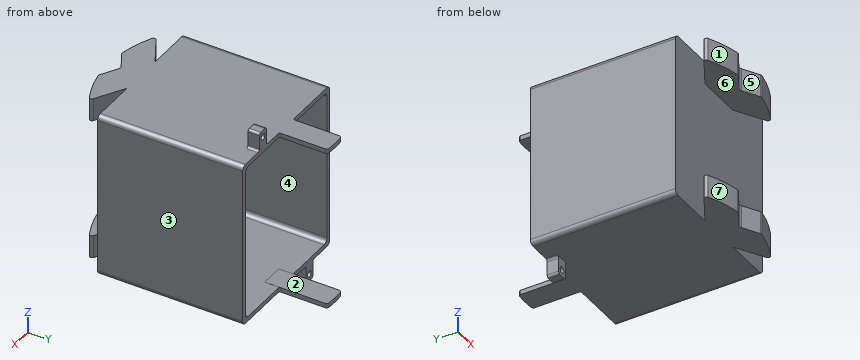
from build123d import *

# Parameters (mm, degrees)
BOSS_EXTRUDE1_DEPTH = 70
CUT_EXTRUDE1_DEPTH  = 79.756
BOSS_EXTRUDE3_DEPTH = 2.54
BOSS_EXTRUDE4_DEPTH = 2.54
BOSS_EXTRUDE5_DEPTH = 12.7
BOSS_EXTRUDE6_START = -2.54
BOSS_EXTRUDE6_DEPTH = 2.54
BOSS_EXTRUDE7_START = -12.7
BOSS_EXTRUDE7_DEPTH = 12.7
BOSS_EXTRUDE8_DEPTH = 8
SKETCH9_R           = 1.685173155
BOSS_EXTRUDE9_DEPTH = 6.35
FILLET1_R           = 1.27
FILLET3_R           = 1


# Read off the part's stored shape, not the designer's step: Boss-Extrude8
with BuildPart() as part:
    # Sketch1 → Boss-Extrude1 (new body)
    with BuildSketch(Plane(origin=(0, 0, 0), x_dir=(1, 0, 0), z_dir=(0, 1, 0))):
        with BuildLine():
            Line((-36.96, -46), (36.96, -46))
            ThreePointArc((36.96, -46), (38.756051224, -45.256051224), (39.5, -43.46))
            Line((39.5, -43.46), (39.5, 43.46))
            ThreePointArc((39.5, 43.46), (38.756051224, 45.256051224), (36.96, 46))
            Line((36.96, 46), (-36.96, 46))
            ThreePointArc((-36.96, 46), (-38.756051224, 45.256051224), (-39.5, 43.46))
            Line((-39.5, 43.46), (-39.5, -43.46))
            ThreePointArc((-39.5, -43.46), (-38.756051224, -45.256051224), (-36.96, -46))
        make_face()
    extrude(amount=-BOSS_EXTRUDE1_DEPTH)

    # Sketch2 → Cut-Extrude1 (cut)
    with BuildSketch(Plane(origin=(0, 0, 0), x_dir=(1, 0, 0), z_dir=(0, 1, 0))):
        with BuildLine():
            Line((-34.46, -43.5), (34.46, -43.5))
            ThreePointArc((34.46, -43.5), (36.256051224, -42.756051224), (37, -40.96))
            Line((37, -40.96), (37, 40.96))
            ThreePointArc((37, 40.96), (36.256051224, 42.756051224), (34.46, 43.5))
            Line((34.46, 43.5), (-34.46, 43.5))
            ThreePointArc((-34.46, 43.5), (-36.256051224, 42.756051224), (-37, 40.96))
            Line((-37, 40.96), (-37, -40.96))
            ThreePointArc((-37, -40.96), (-36.256051224, -42.756051224), (-34.46, -43.5))
        make_face()
    extrude(amount=-CUT_EXTRUDE1_DEPTH, mode=Mode.SUBTRACT)

    # Sketch4 → Boss-Extrude3 (add)
    with BuildSketch(Plane.XZ.offset(70)):
        with BuildLine():
            Line((36.96, 46), (-36.96, 46))
            ThreePointArc((-36.96, 46), (-38.756051224, 45.256051224), (-39.5, 43.46))
            Line((-39.5, 43.46), (-39.5, -43.46))
            ThreePointArc((-39.5, -43.46), (-38.756051224, -45.256051224), (-36.96, -46))
            Line((-36.96, -46), (36.96, -46))
            ThreePointArc((36.96, -46), (38.756051224, -45.256051224), (39.5, -43.46))
            Line((39.5, -43.46), (39.5, 43.46))
            ThreePointArc((39.5, 43.46), (38.756051224, 45.256051224), (36.96, 46))
        make_face()
    extrude(amount=BOSS_EXTRUDE3_DEPTH)

    # Sketch5 → Boss-Extrude4 (add)
    with BuildSketch(Plane.XY.offset(46)):
        with BuildLine():
            Line((6.362854251, 0), (6.362854251, 33.604002981))
            ThreePointArc((6.362854251, 33.604002981), (6.027268312, 34.464102023), (5.197861555, 34.869654381))
            ThreePointArc((5.197861555, 34.869654381), (0, 35.084910085), (-5.197861555, 34.869654381))
            ThreePointArc((-5.197861555, 34.869654381), (-6.027268312, 34.464102023), (-6.362854251, 33.604002981))
            Line((-6.362854251, 33.604002981), (-6.362854251, 0))
            Line((-6.362854251, 0), (6.362854251, 0))
        make_face()
    extrude(amount=-BOSS_EXTRUDE4_DEPTH)

    # Sketch5_4 → Boss-Extrude5 (add)
    with BuildSketch(Plane.XY.offset(46)):
        with BuildLine():
            Line((-12.7, -72.54), (-28.453647637, -81.635372704))
            ThreePointArc((-28.453647637, -81.635372704), (-29.088167479, -82.770144478), (-28.392228001, -83.868320535))
            ThreePointArc((-28.392228001, -83.868320535), (-19.920711126, -87.405365539), (-11.024381507, -89.670890825))
            ThreePointArc((-11.024381507, -89.670890825), (-10.582224591, -89.671469352), (-10.166666729, -89.520423878))
            Line((-10.166666729, -89.520423878), (-1.270072648, -84.383972891))
            ThreePointArc((-1.270072648, -84.383972891), (-9.734e-06, -84.043677417), (1.270036321, -84.384035808))
            Line((1.270036321, -84.384035808), (10.165723413, -89.520550737))
            ThreePointArc((10.165723413, -89.520550737), (10.581295609, -89.671620625), (11.023474349, -89.671052407))
            ThreePointArc((11.023474349, -89.671052407), (19.880019162, -87.418945228), (28.31647684, -83.906602049))
            ThreePointArc((28.31647684, -83.906602049), (29.01385185, -82.810943696), (28.383639864, -81.675324049))
            Line((28.383639864, -81.675324049), (12.7, -72.54))
            Line((12.7, -72.54), (-12.7, -72.54))
        make_face()
    extrude(amount=-BOSS_EXTRUDE5_DEPTH)

    # Sketch6 → Boss-Extrude6 (add)
    with BuildSketch(Plane(origin=(0, 0, -46), x_dir=(-1, 0, 0), z_dir=(0, 0, -1)).offset(BOSS_EXTRUDE6_START)):
        with BuildLine():
            Line((-6.362854251, 0), (-6.362854251, 33.604002981))
            ThreePointArc((-6.362854251, 33.604002981), (-6.027268312, 34.464102023), (-5.197861555, 34.869654381))
            ThreePointArc((-5.197861555, 34.869654381), (0, 35.084910085), (5.197861555, 34.869654381))
            ThreePointArc((5.197861555, 34.869654381), (6.027268312, 34.464102023), (6.362854251, 33.604002981))
            Line((6.362854251, 33.604002981), (6.362854251, 0))
            Line((6.362854251, 0), (-6.362854251, 0))
        make_face()
    extrude(amount=BOSS_EXTRUDE6_DEPTH)

    # Sketch6_3 → Boss-Extrude7 (add)
    with BuildSketch(Plane(origin=(0, 0, -46), x_dir=(-1, 0, 0), z_dir=(0, 0, -1)).offset(BOSS_EXTRUDE7_START)):
        with BuildLine():
            Line((-12.7, -72.54), (12.7, -72.54))
            Line((12.7, -72.54), (28.453647637, -81.635372704))
            ThreePointArc((28.453647637, -81.635372704), (29.088167479, -82.770144478), (28.392228001, -83.868320535))
            ThreePointArc((28.392228001, -83.868320535), (19.920711126, -87.405365539), (11.024381507, -89.670890825))
            ThreePointArc((11.024381507, -89.670890825), (10.582224591, -89.671469352), (10.166666729, -89.520423878))
            Line((10.166666729, -89.520423878), (1.270072648, -84.383972891))
            ThreePointArc((1.270072648, -84.383972891), (9.734e-06, -84.043677417), (-1.270036321, -84.384035808))
            Line((-1.270036321, -84.384035808), (-10.165723413, -89.520550737))
            ThreePointArc((-10.165723413, -89.520550737), (-10.581295609, -89.671620625), (-11.023474349, -89.671052407))
            ThreePointArc((-11.023474349, -89.671052407), (-19.880019162, -87.418945228), (-28.31647684, -83.906602049))
            ThreePointArc((-28.31647684, -83.906602049), (-29.01385185, -82.810943696), (-28.383639864, -81.675324049))
            Line((-28.383639864, -81.675324049), (-12.7, -72.54))
        make_face()
    extrude(amount=BOSS_EXTRUDE7_DEPTH)

    # Boss-Extrude8 outline → Boss-Extrude8 (add)
    with BuildSketch(Plane(origin=(0, 0, 0), x_dir=(1, 0, 0), z_dir=(0, 1, 0))):
        with BuildLine():
            Line((37, 40.96), (37, -40.96))
            ThreePointArc((37, -40.96), (36.257110645, -42.757110645), (34.46, -43.5))
            Line((34.46, -43.5), (6.362854251, -43.5))
            Line((6.362854251, -43.5), (6.362854251, -46))
            Line((6.362854251, -46), (36.96, -46))
            ThreePointArc((36.96, -46), (38.756051224, -45.256051224), (39.5, -43.46))
            Line((39.5, -43.46), (39.5, 43.46))
            ThreePointArc((39.5, 43.46), (38.756051224, 45.256051224), (36.96, 46))
            Line((36.96, 46), (6.362854251, 46))
            Line((6.362854251, 46), (6.362854251, 43.5))
            Line((6.362854251, 43.5), (34.46, 43.5))
            ThreePointArc((34.46, 43.5), (36.256051224, 42.756051224), (37, 40.96))
        make_face()
        with BuildLine():
            Line((-6.362854251, -43.46), (-34.46, -43.5))
            ThreePointArc((-34.46, -43.5), (-36.257110645, -42.757110645), (-37, -40.96))
            Line((-37, -40.96), (-37, 40.96))
            ThreePointArc((-37, 40.96), (-36.256051224, 42.756051224), (-34.46, 43.5))
            Line((-34.46, 43.5), (-6.362854251, 43.5))
            Line((-6.362854251, 43.5), (-6.362854251, 46))
            Line((-6.362854251, 46), (-36.96, 46))
            ThreePointArc((-36.96, 46), (-38.756051224, 45.256051224), (-39.5, 43.46))
            Line((-39.5, 43.46), (-39.5, -43.46))
            ThreePointArc((-39.5, -43.46), (-38.756051224, -45.256051224), (-36.96, -46))
            Line((-36.96, -46), (-6.362854251, -46))
            Line((-6.362854251, -46), (-6.362854251, -43.46))
        make_face()
    extrude(amount=BOSS_EXTRUDE8_DEPTH)

    # Sketch9 → Boss-Extrude9 (add)
    # profile 1 of 2: a face of its own
    with BuildSketch(Plane(origin=(0, 8, 0), x_dir=(1, 0, 0), z_dir=(0, 1, 0))):
        with BuildLine():
            Line((-24.26, 46), (-17.91, 46))
            Line((-17.91, 46), (-17.91, 54.89))
            ThreePointArc((-17.91, 54.89), (-18.281974388, 55.788025612), (-19.18, 56.16))
            Line((-19.18, 56.16), (-22.99, 56.16))
            ThreePointArc((-22.99, 56.16), (-23.888025612, 55.788025612), (-24.26, 54.89))
            Line((-24.26, 54.89), (-24.26, 46))
        make_face()
        with Locations(Location((-21.085, 52.35, 0), (0, 0, 270))):
            Circle(SKETCH9_R, mode=Mode.SUBTRACT)
    # profile 2 of 2: a face of its own
    with BuildSketch(Plane(origin=(0, 8, 0), x_dir=(1, 0, 0), z_dir=(0, 1, 0))):
        with BuildLine():
            Line((24.26, -46), (17.91, -46))
            Line((17.91, -46), (17.91, -54.89))
            ThreePointArc((17.91, -54.89), (18.281974388, -55.788025612), (19.18, -56.16))
            Line((19.18, -56.16), (22.99, -56.16))
            ThreePointArc((22.99, -56.16), (23.888025612, -55.788025612), (24.26, -54.89))
            Line((24.26, -54.89), (24.26, -46))
        make_face()
        with Locations(Location((21.085, -52.35, 0), (0, 0, 90))):
            Circle(SKETCH9_R, mode=Mode.SUBTRACT)
    extrude(amount=-BOSS_EXTRUDE9_DEPTH)

    # Fillet1
    fillet1_edges = [part.edges().sort_by_distance(p)[0] for p in [
        (-17.91, 4.825, -46),
        (-24.26, 4.825, -46),
        (17.91, 4.825, 46),
        (24.26, 4.825, 46),
    ]]
    fillet(fillet1_edges, radius=FILLET1_R)

    # Fillet3
    fillet3_edges = [part.edges().sort_by_distance(p)[0] for p in [
        (6.362854251, 8, 44.75),
        (6.362854251, 8, -44.75),
        (-6.362854251, 8, -44.75),
        (-6.362854251, 8, 44.73),
    ]]
    fillet(fillet3_edges, radius=FILLET3_R)


solid = part.part
Part model, mm, in its own coordinate system. Face numbers are marked on the shaded views. A direction names the side the tool comes from. Coordinates: 2 decimals unless noted, no trailing zeros. Write each loop counter-clockwise with the first axis right and the second up, starting at its lowest first coordinate (ties: lowest second). Pieces come first, ordered by that corner, then holes. Notation, with made-up numbers: (73, 79.25) - (101, 79.25) arc R19 cw to (101, 108.25) - close; hole circle Ø7 at (-12, 55). An arc over 180 degrees is marked (long way). Put each result on its own line as item: value.
1. Band-saw the part on C-C (x = 15). Write the cut outline in (y, z), then the cut area to 3 significant figures.
Final values:
outline: (-88.83, -46) - (-73.88, -46) - (-73.88, -33.3) - (-88.83, -33.3) - close; (-88.83, 33.3) - (-73.88, 33.3) - (-73.88, 46) - (-88.83, 46) - close; (-72.54, -46) - (8, -46) - (8, -43.5) - (-70, -43.5) - (-70, 43.5) - (8, 43.5) - (8, 46) - (-72.54, 46) - close
area: 1,000 mm²
2. Band-saw the part on B-B (y = 11). Write the cut outline in (x, z), then the cut area to 3 significant figures.
Final values:
outline: (-6.36, -46) - (6.36, -46) - (6.36, -43.46) - (-6.36, -43.46) - close; (-6.36, 43.46) - (6.36, 43.46) - (6.36, 46) - (-6.36, 46) - close
area: 64.6 mm²
3. 3-axis set-ups, long thin cutter, end or side, ignore diameter. For the marked faces 5, 6 and 7: which of +Z, -Z, +X, -X, +Y, -Y reach the whole face in a straight line?
Final values:
face 5: +Z, -Z, -Y
face 6: +X, -X, -Y
face 7: +Z, -Z, -X, -Y
4. Flat gauge pins, fed straight in: pin 1 Ø3 at (x, y) = (17, 2.5) entering from +Z; pin 2 Ø0.8 at (x, z) = (35.5, 42.5) entering from +Y; pin 3 Ø10 at (x, z) = (-1.5, 18) entering from -Y. Where does each tip first touch, or does it go through?
Final values:
pin 1: stops at z = 55.96
pin 2: stops at y = -70
pin 3: stops at y = -72.54
5. Probe line 1 along Z through (x, y) = (4.5, -37); line 2 along X through (y, z) = (-10, 7.5); line 3 along X through (y, z) = (6.25, 52.35). List the from-to ranges inside material, lowest first. Write a range as [from, to].
Final values:
line 1: z = [-46, -43.5], [43.5, 46]
line 2: x = [-39.5, -37], [37, 39.5]
line 3: x = [17.91, 19.4], [22.77, 24.26]
6. Band-saw the part on D-D (y = -55.5). Write the cut outline in (x, z).
Final values:
outline: (-39.5, -43.46) arc R2.54 ccw to (-36.96, -46) - (36.96, -46) arc R2.54 ccw to (39.5, -43.46) - (39.5, 43.46) arc R2.54 ccw to (36.96, 46) - (-36.96, 46) arc R2.54 ccw to (-39.5, 43.46) - close; hole (-37, -40.96) arc R2.54 ccw to (-34.46, -43.5) - (34.46, -43.5) arc R2.54 ccw to (37, -40.96) - (37, 40.96) arc R2.54 ccw to (34.46, 43.5) - (-34.46, 43.5) arc R2.54 ccw to (-37, 40.96) - close
7. Two-plate mould, pull along X, no slides. Class the marked faces 1, 2, 3 and 4: +X half, -X half, draft (parallel to the pull), parting line (faces both ways), or undercut.
Final values:
face 1: -X half
face 2: undercut
face 3: +X half
face 4: undercut
8. Band-saw the part on A-A (z = 52.35). Write the cut outline in (x, y), then the cut area to 3 significant figures.
Final values:
outline: (17.91, 1.65) - (19.4, 1.65) - (19.4, 8) - (17.91, 8) - close; (22.77, 1.65) - (24.26, 1.65) - (24.26, 8) - (22.77, 8) - close
area: 18.9 mm²
